Geometry check sheet. Reference: the model listing, model coordinates, mm. Face numbers are marked on the shaded views. A direction names the side the tool comes from. Give positions to 0.01 mm unless a question says otherwise; leave off trailing zeros. Write each loop counter-clockwise with the first axis right and the second up, starting at its lowest first coordinate (ties: lowest second). Pieces come first, ordered by that corner, then holes. Notation, with made-up numbers: M 22.5,73.5 L 47.5,73.5 A6 cw 47.5,77.5 Z; hole C 52,-36.75 d4. An arc over 180 degrees is marked long. One line per item, written item: value. Start each with the question number.
1. Cross-section at B-B on z = 4.5. Record the cut outline in (x, y) (3 decimals).
2. Cross-section at C-C on x = 17. Record the cut outline in (y, z), then the cut area to 3 significant figures.
3. Gauge pin test, flat ends, axial feed: pin 1 (3 mm diameter, centred on x = 1, y = -1.5, fed in from +Z); pin 2 (2 mm diameter, centred on y = 12, z = 6, fed in from -X); pin 3 (12 mm diameter, centred on x = -7, y = 5.5, fed in from -Z). Record the tip position at first contact, or that the pin passes through.
4. Release check for a two-part mould opening along Y. For the marked faces 4, 5, 6 and 7 record: pulls with the +Y half, pulls with the -Y half, needs draft (parallel to the pull), parting line crosses it, or undercut.
5. Cross-section at A-A on y = -12.5. Record the cut outline in (x, z), then the cut area to 3 significant figures.
6. Tool access check on the marked faces 1, 2 and 3. Record the directions out of +Z, -Z, +X, -X, +Y, -Y that give a thin tool (end or side, any length) a straight path to the whole face; none if there is none.
7. Scan lines: line 1 (Y direction, x = 0, z = 29.5); line 2 (Y direction, x = 0.5, z = 2.5); line 3 (Z direction, x = 18, y = -3.5). Record each from-to range of solid material in increasing order.
from build123d import *

# Parameters (mm, degrees)
F3_DEPTH = 14.097
F4_R     = 4.7625
F5_DEPTH = 9.525


with BuildPart() as f1:
    # F0 (on Front) → F1 (revolve)
    with BuildSketch(Plane.XZ):
        Polygon((6.35, 24.5250865847), (6.35, 34.0500865847), (0, 34.0500865847), (0, -10.3999134153), (6.35, 0), (22.225, 0), (22.225, 9.0132579207), (8.8899998294, 9.0132579207), align=None)
    revolve(axis=Axis((0, 0, 11.8250865847), (0, 0, 1)))

    # F2 (on Top) → F3 (cut)
    with BuildSketch(Plane.XY):
        with BuildLine():
            ThreePointArc((-14.113121628, -17.1688794892), (0.2443956371, -22.2236562197), (14.487278372, -16.8543582011))
            ThreePointArc((14.487278372, -16.8543582011), (12.207059324, -13.6802064233), (11.8003316443, -9.7931495662))
            Line((11.8003316443, -9.7931495662), (6.0394839652, -6.5235522098))
            ThreePointArc((6.0394839652, -6.5235522098), (0.0488798663, -8.889865621), (-5.9673830231, -6.5895705365))
            Line((-5.9673830231, -6.5895705365), (-11.470085079, -9.7931648991))
            ThreePointArc((-11.470085079, -9.7931648991), (-11.8071714813, -13.8337865787), (-14.113121628, -17.1688794892))
        make_face()
        with BuildLine():
            ThreePointArc((21.8983417722, -3.7964789779), (22.1431848532, -1.9052531477), (22.225, 0))
            ThreePointArc((22.225, 0), (18.1777280494, 12.7875262644), (7.5099648628, 20.9177210221))
            ThreePointArc((7.5099648628, 20.9177210221), (5.9196955053, 17.4232913204), (2.8274223411, 15.1478040653))
            Line((2.8274223411, 15.1478040653), (2.8274223411, 8.4283914779))
            ThreePointArc((2.8274223411, 8.4283914779), (7.2169205556, 5.1911614976), (8.89, 0))
            ThreePointArc((8.89, 0), (8.8417204308, -0.9252458182), (8.6974061138, -1.8404420369))
            Line((8.6974061138, -1.8404420369), (14.4582537929, -5.1100393933))
            ThreePointArc((14.4582537929, -5.1100393933), (18.0040397888, -3.4662510593), (21.8983417722, -3.7964789779))
        make_face()
        with BuildLine():
            ThreePointArc((-2.5544860487, 15.0469797465), (-5.8234880662, 17.3140797385), (-7.5044304492, 20.9197071833))
            ThreePointArc((-7.5044304492, 20.9197071833), (-19.2055517537, 11.1846952054), (-21.8983417722, -3.7964789779))
            ThreePointArc((-21.8983417722, -3.7964789779), (-17.8595819955, -3.4377725991), (-14.1793440119, -5.1395655315))
            Line((-14.1793440119, -5.1395655315), (-8.676641956, -1.9359711689))
            ThreePointArc((-8.676641956, -1.9359711689), (-7.6707699458, 4.4934828851), (-2.5544860487, 8.5150866717))
            Line((-2.5544860487, 8.5150866717), (-2.5544860487, 15.0469797465))
        make_face()
    extrude(amount=F3_DEPTH, mode=Mode.SUBTRACT)

    # F4 (on face) → F5 (cut)
    with BuildSketch(Plane.XY.offset(34.0500865847)):
        Circle(F4_R)
    extrude(amount=-F5_DEPTH, mode=Mode.SUBTRACT)


solid = f1.part
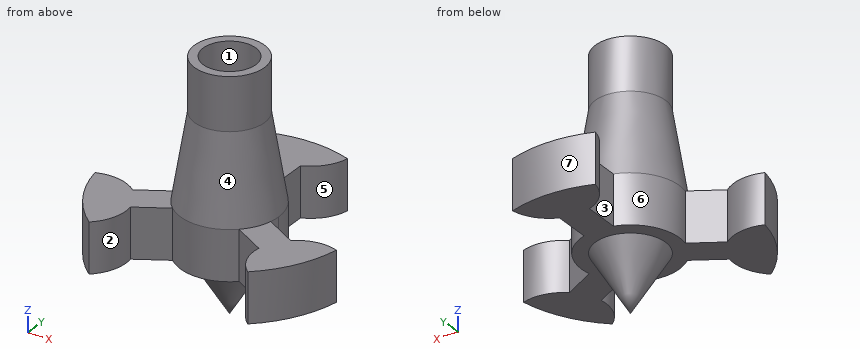
Report:
1. outline: M -21.898,-3.796 A22.225 ccw -14.113,-17.169 A7.861 ccw -11.47,-9.793 L -5.967,-6.59 A8.89 ccw 6.039,-6.524 L 11.8,-9.793 A7.62 ccw 14.487,-16.854 A22.225 ccw 21.898,-3.796 A7.62 ccw 14.458,-5.11 L 8.697,-1.84 A8.89 ccw 2.827,8.428 L 2.827,15.148 A7.62 ccw 7.51,20.918 A22.225 ccw -7.504,20.92 A7.62 ccw -2.554,15.047 L -2.554,8.515 A8.89 ccw -8.677,-1.936 L -14.179,-5.14 A7.861 ccw Z
2. outline: M -14.32,0 L -3.71,0 L -3.71,9.01 L -14.32,9.01 Z
2. area: 95.6 mm^2
3. pin 1: stops at z = 24.53
3. pin 2: stops at x = -2.55
3. pin 3: stops at z = -5.65
4. face 4: parting line crosses it
4. face 5: undercut
4. face 6: undercut
4. face 7: pulls with the +Y half
5. outline: M -18.38,0 L -11.46,0 L -11.46,9.01 L -18.38,9.01 Z; M 11.86,0 L 18.38,0 L 18.38,9.01 L 11.86,9.01 Z
5. area: 121 mm^2
6. face 1: +Z
6. face 2: +Z, -Z
6. face 3: +Z, -Z, -X
7. line 1: y = -6.35 to -4.76, 4.76 to 6.35
7. line 2: y = -8.88 to 22.22
7. line 3: z = 0 to 9.01
